```python
from build123d import *

# Parameters (mm, degrees)
CROQUIS1_W              = 26
CROQUIS1_H              = 28.884781413
CROQUIS1_R              = 8
SALIENTE_EXTRUIR1_DEPTH = 3
CROQUIS2_W              = 30
CROQUIS2_H              = 32.884781413
SALIENTE_EXTRUIR2_DEPTH = 5
SALIENTE_EXTRUIR3_DEPTH = 5
CROQUIS5_R              = 8
CORTAR_EXTRUIR1_DEPTH   = 10


with BuildPart() as part:
    # Croquis1 → Saliente-Extruir1 (new body)
    with BuildSketch(Plane.XY):
        with Locations((11, 9.157609294)):
            Rectangle(CROQUIS1_W, CROQUIS1_H)
        with Locations((11, 9.157609293)):
            Circle(CROQUIS1_R, mode=Mode.SUBTRACT)
    extrude(amount=SALIENTE_EXTRUIR1_DEPTH)

    # Croquis2 → Saliente-Extruir2 (add)
    with BuildSketch(Plane.XY.offset(3)):
        with Locations((11, 9.157609294)):
            Rectangle(CROQUIS2_W, CROQUIS2_H)
    extrude(amount=SALIENTE_EXTRUIR2_DEPTH)

    # Croquis4 → Saliente-Extruir3 (add)
    with BuildSketch(Plane.XY.offset(8)):
        Polygon((-9, 14.157609293), (-9, 4.157609293), (-4, 6.657609293), (-4, 11.657609293), align=None)
    extrude(amount=-SALIENTE_EXTRUIR3_DEPTH)

    # Croquis5 → Cortar-Extruir1 (cut)
    with BuildSketch(Plane(origin=(0, 0, 3), x_dir=(-1, 0, 0), z_dir=(0, 0, -1))):
        with Locations((-11, 9.157609293)):
            Circle(CROQUIS5_R)
    extrude(amount=-CORTAR_EXTRUIR1_DEPTH, mode=Mode.SUBTRACT)


solid = part.part
```
Read the model definition and answer for the solid it produces. Units are mm, in the model's axes. A direction names the side the tool comes from. Give positions to 0.01 mm unless a question says otherwise; leave off trailing zeros. Order: outer loops, then holes, each group sorted by start corner. A loop starts at its lowest first (then second) coordinate and runs counter-clockwise, first axis right, second up.
(1) Find section D-D (y = 11). Give the vertices of the cut face in (x, z).
(2) For faces 4 (the flat face through (11, 23.6, 1)), 5 (the flat face through (11, -5.285, 1)), 6 (the flat face through (-6.465, 12.89, 5.535)), 7 (the flat face through (-6.535, 5.39, 5.535)), 8 (the flat face through (24, 9, 1)), determine the directions among +Z, -Z, +X, -X, +Y, -Y from which every point of the face is accessible in a straight line to the end or side of a thin tool.
(3) Find section A-A (x = 11). Give the vertices of the cut face in (y, z), plus the area to 3 significant figures.
(4) Find section C-C (z = 6). Give the vertices of the cut face in (x, y), plus the area to 3 significant figures.
(5) Straight lines are drawn through the part: L1, parallel to X at y = 9, z = 4.25; L2, parallel to Y at x = 11, z = 0.75; L3, parallel to Y at x = 11, z = 4.7. For each, find the intervals that lie inside material, in ascending order.
(6) Find section B-B (y = 19.5). Give the vertices of the cut face in (x, z), plus the area to 3 significant figures.
(7) For a pull along X with two mould halves and no side action, classify faces 1 (the flat face through (-2, 9, 1)), 2 (the flat face through (-3, 9, 3)), 3 (the flat face through (-4, 19, 5)) as released by +X, released by -X, zero draft, split by the parting line, or undercut.
(8) Given pin 1 (3.5 mm diameter, centred on x = 12.5, z = 1.5, fed in from -Y); pin 2 (1.5 mm diameter, centred on x = 12.5, z = 2, fed in from +Y); pin 3 (1.5 mm diameter, centred on y = 10, z = 1.5, fed in from -X); pin 4 (1.5 mm diameter, centred on y = -2.5, z = 5, fed in from -X), each flat-ended and moving along its own axis, determine where each tip first touches the part or whether it passes through.
Result sheet:
1. outline: (-9, 3) - (-2, 3) - (-2, 0) - (3.22, 0) - (3.22, 8) - (-9, 8) - close; (18.78, 0) - (24, 0) - (24, 3) - (26, 3) - (26, 8) - (18.78, 8) - close
2. face 4: -Z, +X, -X, +Y
2. face 5: -Z, +X, -X, -Y
2. face 6: +Z, -Z, +Y
2. face 7: +Z, -Z, -Y
2. face 8: -Z, +X, +Y, -Y
3. outline: (-7.28, 3) - (-5.28, 3) - (-5.28, 0) - (1.16, 0) - (1.16, 8) - (-7.28, 8) - close; (17.16, 0) - (23.6, 0) - (23.6, 3) - (25.6, 3) - (25.6, 8) - (17.16, 8) - close
3. area: 123 mm2
4. outline: (-9, 4.16) - (-4, 6.66) - (-4, -7.28) - (26, -7.28) - (26, 25.6) - (-4, 25.6) - (-4, 11.66) - (-9, 14.16) - close; hole circle Ø16 at (11, 9.16)
4. area: 823 mm2
5. L1: x = -9 to 3, 19 to 26
5. L2: y = -5.28 to 1.16, 17.16 to 23.6
5. L3: y = -7.28 to 1.16, 17.16 to 25.6
6. outline: (-4, 3) - (-2, 3) - (-2, 0) - (24, 0) - (24, 3) - (26, 3) - (26, 8) - (-4, 8) - close
6. area: 228 mm2
7. face 1: released by -X
7. face 2: zero draft
7. face 3: undercut
8. pin 1: stops at y = -7.28
8. pin 2: stops at y = 23.6
8. pin 3: stops at x = -2
8. pin 4: stops at x = -4
